Autodesk Inventor part; units mm, degrees
ref_plane "YZ Plane" through (0, 0, 0) normal (1, 0, 0) x (0, 1, 0)
ref_plane "XZ Plane" through (0, 0, 0) normal (0, 1, 0) x (-1, 0, 0)
ref_plane "XY Plane" through (0, 0, 0) normal (0, 0, 1) x (1, 0, 0)
sketch "Szkic1" plane through (0, 0, 0) normal (0, 1, 0) x (-1, 0, 0)
  line L0 (-65, 0) -> (-73, 0)
  line L1 (-73, 0) -> (-73, -132.5)
  line L2 (-73, -132.5) -> (-25, -132.5)
  line L3 (0, -107.5) -> (0, -65)
  arc A0 (-25, -132.5) -> (0, -107.5) centre (-25, -107.5) ccw
  arc A1 (0, -65) -> (-65, 0) centre (-65, -65) ccw
  circle A2 centre (-73, -37.5) radius 37.5
  point P0 (0, 0)
  point P1 (0, -132.5)
  point P2 (-73, -75)
  dimension "d4" = 75
  dimension "d0" = 73
  dimension "d1" = 132.5
  dimension "d2" = 25
  dimension "d3" = 65
extrude "Wyciągnięcie proste1" add sketch "Szkic1" along normal blind 16 contours A1 L3 A0 L2 L1 A2 L0
sketch "Szkic2" plane through (0, 0, 0) normal (0, -1, 0) x (1, 0, 0)
  arc A0 (73, 0) -> (73, -75) centre (73, -37.5) ccw
  circle A1 centre (73, -37.5) radius 37.5
  point P0 (0, 0)
  point P1 (73, -75)
extrude "Wyciągnięcie proste2" add sketch "Szkic2" against normal blind 63
sketch "Szkic3" plane through (0, 16, 0) normal (0, 1, 0) x (1, 0, 0)
  arc A0 (25, 132.5) -> (0, 107.5) centre (25, 107.5) ccw
  line L0 (73, 132.5) -> (25, 132.5)
  line L1 (73, 75) -> (73, 132.5)
  line L2 (73, 132.5) -> (73, 75)
  line L3 (73, 132.5) -> (57, 132.5)
  line L4 (57, 132.5) -> (57, 71.4153)
  arc A1 (73, 75) -> (73, 0) centre (73, 37.5) ccw
  arc A2 (73, 75) -> (57, 71.4153) centre (73, 37.5) ccw
  point P0 (0, 0)
  dimension "d9" = 16
extrude "Wyciągnięcie proste3" add sketch "Szkic3" along normal blind 47
fillet "Zaokrąglenie1" radius 25 1 edges at (65, 63, -132.5)
sketch "Szkic4" plane through (0, 63, 0) normal (0, 1, 0) x (1, 0, 0)
  arc A0 (57, 71.4153) -> (73, 0) centre (73, 37.5) ccw
  point P0 (0, 0)
hole "Otwór1" at (73, 63, -37.5) direction (0, -1, 0) diameter 50 end through all
sketch "Szkic5" plane through (57, 16, -132.5) normal (-1, 0, 0) x (0, 0, 1)
  arc A0 (25, 47) -> (0, 22) centre (25, 22) ccw
  point P0 (132.5, -16)
hole "Otwór2" at (57, 38, -107.5) direction (1, 0, 0) diameter 20 end through all
sketch "Szkic6" plane through (0, 16, 0) normal (0, 1, 0) x (1, 0, 0)
  arc A0 (25, 132.5) -> (0, 107.5) centre (25, 107.5) ccw
  point P0 (0, 0)
hole "Otwór3" at (25, 16, -107.5) direction (0, -1, 0) diameter 22 end through all
Can you work these out from the model? Positions are in its coordinate system, mm. A direction names the side the tool comes from. Round coordinates to 2 decimals unless told otherwise and drop trailing zeros. Write each loop counter-clockwise with the first axis right and the second up, starting at its lowest first coordinate (ties: lowest second). Pieces come first, ordered by that corner, then holes. Notation, with made-up numbers: M 27.25,63.5 L 56.25,63.5 A24 ccw 56.25,91.5 Z; hole C -27,-11.75 d7. An arc over 180 degrees is marked long. Use CSV: the item, a comma, the result in double quotes.
(1) We'd pull the mould along X, two halves only. Please class faces 4 (the flat face through (73, 31, -97)), 5 (the cylindrical face through (24.52, 7.89, -118.49)), 6 (the flat face through (29, 16, -80)): +X half, -X half, draft (parallel to the pull), parting line (faces both ways), or undercut.
Check values:
face 4,"+X half"
face 5,"undercut"
face 6,"draft"
(2) I need wall thicknesses on line 1 along Z through (x, y) = (74, 17); line 2 along X through (y, z) = (7.5, -107.5); line 3 along Y through (x, z) = (68.5, -107.5). Which ranges of each line are inside material? Lowest first, please.
Check values:
line 1,"-74.99 to -62.48, -12.52 to -0.01"
line 2,"0 to 14, 36 to 73"
line 3,"0 to 28, 48 to 63"
(3) Imagine slicing it at B-B (x = 21.5). Write out the boundary of the cut face in (y, z).
Check values:
outline,"M 0,-132.25 L 16,-132.25 L 16,-117.93 L 0,-117.93 Z; M 0,-97.07 L 16,-97.07 L 16,-16.7 L 0,-16.7 Z"
(4) Imagine slicing it at D-D (z = -91). Write out the boundary of the cut face in (x, y), plus the area to 3 significant figures.
Check values:
outline,"M 0,0 L 73,0 L 73,63 L 57,63 L 57,16 L 0,16 Z"
area,"1,920 mm^2"
(5) On a 3-axis mill with a long thin cutter (end or side, diameter ignored), from which of +Z, -Z, +X, -X, +Y, -Y can I reach the whole of each face in a straight line? I mean faces 1 (the flat face through (69, 8, 0)), 2 (the flat face through (57, 39, -96)), 3 (the cylindrical face through (102.62, 31.06, -14.5)). Say none if no direction works.
Check values:
face 1,"+Z, +X, -X, +Y, -Y"
face 2,"-Z, -X, +Y"
face 3,"+Y"
(6) I'm going to push flat-ended pins straight in: pin 1 (4 mm diameter, centred on x = 63, y = 24.5, fed in from +Z); pin 2 (1.5 mm diameter, centred on y = 9.5, z = -20, fed in from -X); pin 3 (20 mm diameter, centred on x = 25, z = -107.5, fed in from -Y); pin 4 (10 mm diameter, centred on y = 44.5, z = -72.5, fed in from -X). Where does each tip first touch, or does it pass through?
Check values:
pin 1,"z = -0.86"
pin 2,"x = 17.39"
pin 3,"through"
pin 4,"x = 50.5"
(7) Imagine slicing it at C-C (z = -37.5). Write out the boundary of the cut face in (x, y).
Check values:
outline,"M 6.1,0 L 48,0 L 48,63 L 35.5,63 L 35.5,16 L 6.1,16 Z; M 98,0 L 110.5,0 L 110.5,63 L 98,63 Z"
(8) Imagine slicing it at A-A (y = 36). Write out the boundary of the cut face in (x, z), plus the area to 3 significant figures.
Check values:
outline,"M 57,-132.5 L 73,-132.5 L 73,-117.3 L 57,-117.3 Z; M 57,-97.7 L 73,-97.7 L 73,-75 A37.5 ccw long 57,-71.42 Z; hole C 73,-37.5 d50"
area,"3,080 mm^2"
